from build123d import *

# Parameters (mm, degrees)
F0_W      = 965.2
F0_H      = 101.6
F1_DEPTH  = 6.35
F2_W      = 88.9
F2_H      = 38.1
F3_DEPTH  = 304.8
F4_W      = 88.9
F4_H      = 38.1
F5_DEPTH  = 88.9
F6_W      = 38.1
F6_H      = 88.9
F7_DEPTH  = 101.6
F8_W      = 88.9
F8_H      = 38.1
F9_DEPTH  = 88.9
F10_W     = 38.1
F10_H     = 88.9
F11_DEPTH = 101.6
F13_DEPTH = 6.35


with BuildPart() as f1:
    # F0 (on Front) → F1 (new body)
    with BuildSketch(Plane.XZ):
        Rectangle(F0_W, F0_H)
    extrude(amount=F1_DEPTH)

    # F2 (on face) → F3 (join)
    with BuildSketch(Plane.XZ.offset(6.35)):
        with Locations((-387.35, -31.75)):
            Rectangle(F2_W, F2_H)
        with Locations((387.35, -31.75)):
            Rectangle(F2_W, F2_H)
    extrude(amount=F3_DEPTH)

    # F4 (on face) → F5 (join)
    with BuildSketch(Plane(origin=(-431.8, 0, 0), x_dir=(0, -1, 0), z_dir=(-1, 0, 0))):
        with Locations((158.75, -31.75)):
            Rectangle(F4_W, F4_H)
    extrude(amount=F5_DEPTH)

    # F6 (on face) → F7 (join)
    with BuildSketch(Plane.XY.offset(-12.7)):
        with Locations((-501.65, -158.75)):
            Rectangle(F6_W, F6_H)
    extrude(amount=F7_DEPTH)

    # F8 (on face) → F9 (join)
    with BuildSketch(Plane.YZ.offset(431.8)):
        with Locations((-158.75, -31.75)):
            Rectangle(F8_W, F8_H)
    extrude(amount=F9_DEPTH)

    # F10 (on face) → F11 (join)
    with BuildSketch(Plane.XY.offset(-12.7)):
        with Locations((501.65, -158.75)):
            Rectangle(F10_W, F10_H)
    extrude(amount=F11_DEPTH)

    # F12 (on face) → F13 (join)
    with BuildSketch(Plane.XZ.offset(311.15)):
        Polygon((-482.6, -50.8), (-431.8, -50.8), (482.6, -50.8), (482.6, 50.8), (-482.6, 50.8), align=None)
    extrude(amount=F13_DEPTH)


solid = f1.part
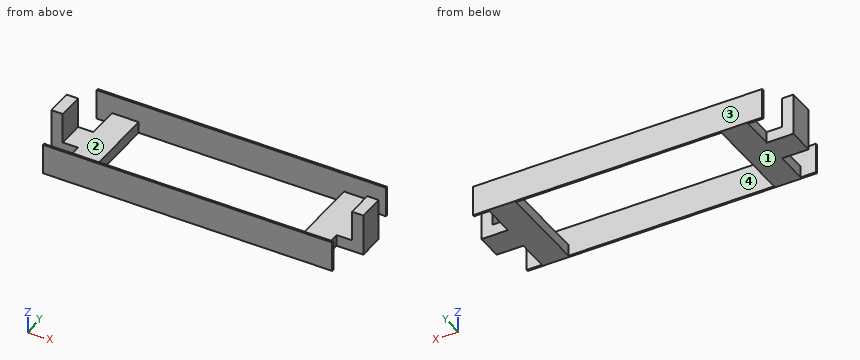
Read the model definition and answer for the solid it produces. Units are mm, in the model's axes. Face numbers are marked on the shaded views. A direction names the side the tool comes from. Round coordinates to 2 decimals unless told otherwise and drop trailing zeros. Loops run counter-clockwise (first coordinate to the right, second up) from the corner with the lowest first, then second, coordinate; pieces in that order, holes last.
Q1. Determine the mould class of the marked faces 3 and 4 for opening direction X: released by +X, released by -X, zero draft, split by the parting line, or undercut.
Q2. Section C-C on z = 21 is taken. Write down the section's boundary in (x, y), and give its area (3 significant figures).
Q3. Each of these flat-tipped pins is pushed along its axis until it touches: pin 1 (3 mm diameter, centred on x = -16, y = -4, fed in from +Z); pin 2 (7 mm diameter, centred on y = -313, z = -24.5, fed in from +X); pin 3 (3 mm diameter, centred on y = -314, z = -19.5, fed in from -X); pin 4 (1.5 mm diameter, centred on x = 68.5, z = 44.5, fed in from +Y). Where does it stop, or does it pass through?
Q4. Consider probe 1 along Y at (x, z) = (-224, 33); probe 2 along X at (y, z) = (-175.5, 3); probe 3 along X at (y, z) = (-89.5, -26). Determine where each line is inside the solid, lowest interval first.
Q5. Which of the six approach directions +Z, -Z, +X, -X, +Y, -Y give full straight-line access (tool end or side, diameter ignored) to the marked faces 1 and 2?
Q6. Section A-A on y = -37 is taken. Write down the section's boundary in (x, z), and give its area (3 significant figures).
Q7. Section B-B on x = 100.5 is taken. Write down the section's boundary in (y, z), and give its area (3 significant figures).
Q8. Section D-D on x = 392.5 is taken. Write down the section's boundary in (y, z), and give its area (3 significant figures).
Output:
1. face 3: zero draft
1. face 4: undercut
2. outline: (-520.7, -203.2) - (-482.6, -203.2) - (-482.6, -114.3) - (-520.7, -114.3) - close; (-482.6, -317.5) - (482.6, -317.5) - (482.6, -311.15) - (-482.6, -311.15) - close; (-482.6, -6.35) - (482.6, -6.35) - (482.6, 0) - (-482.6, 0) - close; (482.6, -203.2) - (520.7, -203.2) - (520.7, -114.3) - (482.6, -114.3) - close
2. area: 19,000 mm2
3. pin 1: stops at z = 50.8
3. pin 2: stops at x = 482.6
3. pin 3: stops at x = -482.6
3. pin 4: stops at y = 0
4. probe 1: y = -317.5 to -311.15, -6.35 to 0
4. probe 2: x = -520.7 to -482.6, 482.6 to 520.7
4. probe 3: x = -431.8 to -342.9, 342.9 to 431.8
5. face 1: -Z, +X, -X, +Y, -Y
5. face 2: +Z
6. outline: (-431.8, -50.8) - (-342.9, -50.8) - (-342.9, -12.7) - (-431.8, -12.7) - close; (342.9, -50.8) - (431.8, -50.8) - (431.8, -12.7) - (342.9, -12.7) - close
6. area: 6,770 mm2
7. outline: (-317.5, -50.8) - (-311.15, -50.8) - (-311.15, 50.8) - (-317.5, 50.8) - close; (-6.35, -50.8) - (0, -50.8) - (0, 50.8) - (-6.35, 50.8) - close
7. area: 1,290 mm2
8. outline: (-317.5, -50.8) - (0, -50.8) - (0, 50.8) - (-6.35, 50.8) - (-6.35, -12.7) - (-311.15, -12.7) - (-311.15, 50.8) - (-317.5, 50.8) - close
8. area: 12,900 mm2
